from build123d import *

# Parameters (mm, degrees)
SKETCH1_R           = 2.25
BOSS_EXTRUDE1_DEPTH = 8
SKETCH2_R           = 1
CUT_EXTRUDE1_DEPTH  = 10
SKETCH3_W           = 12
SKETCH3_H           = 4
SKETCH4_R           = 2.25
BOSS_EXTRUDE2_DEPTH = 4
SKETCH5_R           = 4
CUT_EXTRUDE2_DEPTH  = 4


with BuildPart() as part:
    # Sketch1 → Boss-Extrude1 (new body)
    with BuildSketch(Plane(origin=(0, 0, 0), x_dir=(1, 0, 0), z_dir=(0, 1, 0))):
        with BuildLine():
            Line((-5.822585081, 1.448275862), (-2.426077117, 15.103448276))
            ThreePointArc((-2.426077117, 15.103448276), (0, 17), (2.426077117, 15.103448276))
            Line((2.426077117, 15.103448276), (5.822585081, 1.448275862))
            ThreePointArc((5.822585081, 1.448275862), (6, 0), (5.822585081, -1.448275862))
            Line((5.822585081, -1.448275862), (2.426077117, -15.103448276))
            ThreePointArc((2.426077117, -15.103448276), (0, -17), (-2.426077117, -15.103448276))
            Line((-2.426077117, -15.103448276), (-5.822585081, -1.448275862))
            ThreePointArc((-5.822585081, -1.448275862), (-6, 0), (-5.822585081, 1.448275862))
        make_face()
        with Locations(Location((0, 0, 0), (0, 0, 270))):
            Circle(SKETCH1_R, mode=Mode.SUBTRACT)
    extrude(amount=BOSS_EXTRUDE1_DEPTH)

    # Sketch2 → Cut-Extrude1 (cut)
    with BuildSketch(Plane.XZ):
        with Locations(Location((0, -14.45, 0), (0, 0, 270))):
            Circle(SKETCH2_R)
        with Locations(Location((0, 14.45, 0), (0, 0, 90))):
            Circle(SKETCH2_R)
    extrude(amount=-CUT_EXTRUDE1_DEPTH, mode=Mode.SUBTRACT)

    # Sketch3 → Cut-Revolve1 (revolve, cut)
    with BuildSketch(Plane(origin=(0, 0, 0), x_dir=(0, 0, -1), z_dir=(1, 0, 0)), mode=Mode.PRIVATE) as cut_revolve1_sk:
        with Locations((12, 2)):
            Rectangle(SKETCH3_W, SKETCH3_H)
    revolve(cut_revolve1_sk.sketch.rotate(Axis((0, 0, 0), (0, 1, 0)), 76.032037325), axis=Axis((0, 0, 0), (0, 1, 0)), mode=Mode.SUBTRACT)

    # Sketch4 → Boss-Extrude2 (add)
    with BuildSketch(Plane(origin=(0, 8, 0), x_dir=(1, 0, 0), z_dir=(0, 1, 0))):
        with BuildLine():
            Line((50, 4), (5.187884098, 4))
            Line((5.187884098, 4), (5.187884098, -4))
            Line((5.187884098, -4), (50, -4))
            ThreePointArc((50, -4), (54, 0), (50, 4))
        make_face()
        with Locations(Location((50, 0, 0), (0, 0, 270))):
            Circle(SKETCH4_R, mode=Mode.SUBTRACT)
    extrude(amount=-BOSS_EXTRUDE2_DEPTH)

    # Sketch5 → Cut-Extrude2 (cut)
    with BuildSketch(Plane(origin=(0, 8, 0), x_dir=(1, 0, 0), z_dir=(0, 1, 0))):
        with Locations(Location((0, 0, 0), (0, 0, 270))):
            Circle(SKETCH5_R)
    extrude(amount=-CUT_EXTRUDE2_DEPTH, mode=Mode.SUBTRACT)


solid = part.part
Work out the finished part from the listing and answer in its coordinate system (mm). A direction names the side the tool comes from. Round coordinates to 2 decimals unless told otherwise and drop trailing zeros. Loops run counter-clockwise (first coordinate to the right, second up) from the corner with the lowest first, then second, coordinate; pieces in that order, holes last. Notation, with made-up numbers: M 58.25,61 L 94.25,61 A13 cw 94.25,83 Z; hole C 44.5,43 d9. An arc over 180 degrees is marked long. One line per question, with ' | ' between items. Start each with the question number.
(1) A cutting plane is placed at B-B on x = 0. Write down the section's boundary in (y, z).
(2) Flat-ended cylindrical pins translate along their axes: pin 1 Ø3.5 at (x, z) = (0, 0) entering from -Y; pin 2 Ø7 at (x, z) = (50, 0) entering from -Y; pin 3 Ø2 at (x, y) = (27.5, 7) entering from +Z; pin 4 Ø4.5 at (x, y) = (26, 7) entering from -Z. Find the tip coordinate at first contact, or state that the pin passes through.
(3) Find the intervals of material crossed by line 1 (X direction, y = 5.4, z = 0); line 2 (Z direction, x = 0, y = 3.15); line 3 (X direction, y = 6.8, z = 14.45), in increasing order.
(4) For a pull along X with two mould halves and no side action, classify faces 1 (the face through (0.676, 1.972, 2.146)), 2 (the face through (3.826, 5.972, 9.474)), 3 (the face through (27, 6, 4)), 4 (the face through (-2, 4, 2)) as released by +X, released by -X, zero draft, split by the parting line, or undercut.
(5) A cutting plane is placed at C-C on y = 7.25. Write down the section's boundary in (x, z).
(6) A cutting plane is placed at D-D on z = 14.5. Write down the section's boundary in (x, y).
(7) A tool of negligible diameter and unlimited length cuts with its end or side. For faces 5 (the face through (28, 6, -4)), 6 (the face through (0, 6, -17)), 7 (the face through (-3.905, 6.028, -0.867)), from which of +Z, -Z, +X, -X, +Y, -Y can it reach the whole face along a straight path? Write none if from no direction.
(8) A cutting plane is placed at A-A on z = 0. Write down the section's boundary in (x, y).
Geometry check:
1) outline: M 0,-6 L 4,-6 L 4,-13.45 L 8,-13.45 L 8,-4 L 4,-4 L 4,-2.25 L 0,-2.25 Z; M 0,2.25 L 4,2.25 L 4,4 L 8,4 L 8,13.45 L 4,13.45 L 4,6 L 0,6 Z; M 4,-17 L 8,-17 L 8,-15.45 L 4,-15.45 Z; M 4,15.45 L 8,15.45 L 8,17 L 4,17 Z
2) pin 1: passes through | pin 2: stops at y = 4 | pin 3: stops at z = 4 | pin 4: stops at z = -4
3) line 1: x = -6 to -4, 4 to 47.75, 52.25 to 54 | line 2: z = -6 to -2.25, 2.25 to 6 | line 3: x = -2.59 to -1, 1 to 2.59
4) face 1: undercut | face 2: released by +X | face 3: zero draft | face 4: undercut
5) outline: M -5.82,-1.45 L -2.43,-15.1 A2.5 ccw 2.43,-15.1 L 5.19,-4 L 50,-4 A4 ccw 50,4 L 5.19,4 L 2.43,15.1 A2.5 ccw -2.43,15.1 L -5.82,1.45 A6 ccw Z; hole C 0,0 d8; hole C 0,-14.45 d2; hole C 0,14.45 d2; hole C 50,0 d4.5
6) outline: M -2.58,4 L -1,4 L -1,8 L -2.58,8 Z; M 1,4 L 2.58,4 L 2.58,8 L 1,8 Z
7) face 5: -Z, +X, +Y, -Y | face 6: -Z, +Y, -Y | face 7: +Y
8) outline: M -6,0 L -2.25,0 L -2.25,4 L -4,4 L -4,8 L -6,8 Z; M 2.25,0 L 6,0 L 6,4 L 47.75,4 L 47.75,8 L 4,8 L 4,4 L 2.25,4 Z; M 52.25,4 L 54,4 L 54,8 L 52.25,8 Z
